The listing builds one solid part. Answer for the finished solid, in the listing's coordinates (mm). A direction names the side the tool comes from. Give positions to 0.01 mm unless a question says otherwise; leave off trailing zeros. Write each loop counter-clockwise with the first axis right and the second up, starting at its lowest first coordinate (ties: lowest second). Pieces come first, ordered by that corner, then holes.
```python
from build123d import *

# Parameters (mm, degrees)
ESQUISSE1_R             = 6.75
ESQUISSE1_R_2           = 15
BOSS_EXTRU_1_DEPTH      = 10
ENL_V_MAT_EXTRU_1_DEPTH = 10
CHANFREIN1_SIZE         = 40


with BuildPart() as part:
    # Esquisse1 → Boss.-Extru.1 (new body)
    with BuildSketch(Plane(origin=(0, 0, 0), x_dir=(1, 0, 0), z_dir=(0, 1, 0))):
        Polygon((0, 0), (0, 250), (240, 250), (320, 250), (560, 250), (640, 250), (880, 250), (880, 0), (880, -140), (780, -140), (780, -130), (620, -130), (620, -140), (520, -140), (520, -130), (360, -130), (360, -140), (260, -140), (260, -130), (100, -130), (100, -140), (0, -140), align=None)
        with Locations(Location((480, 20, 0), (0, 0, 270))):
            Circle(ESQUISSE1_R, mode=Mode.SUBTRACT)
        with Locations(Location((400, 20, 0), (0, 0, 270))):
            Circle(ESQUISSE1_R, mode=Mode.SUBTRACT)
        with Locations(Location((400, 80, 0), (0, 0, 270))):
            Circle(ESQUISSE1_R, mode=Mode.SUBTRACT)
        with Locations(Location((480, 80, 0), (0, 0, 270))):
            Circle(ESQUISSE1_R, mode=Mode.SUBTRACT)
        with Locations(Location((280, 190, 0), (0, 0, 270))):
            Circle(ESQUISSE1_R_2, mode=Mode.SUBTRACT)
        with Locations(Location((600, 190, 0), (0, 0, 270))):
            Circle(ESQUISSE1_R_2, mode=Mode.SUBTRACT)
    extrude(amount=BOSS_EXTRU_1_DEPTH)

    # Esquisse2 → Enlèv. mat.-Extru.1 (cut)
    with BuildSketch(Plane(origin=(0, 10, 0), x_dir=(1, 0, 0), z_dir=(0, 1, 0))):
        Polygon((800, 130), (600, 130), (560, 90), (560, -50), (580, -70), (800, -70), (820, -50), (820, 110), align=None)
        Polygon((80, 130), (60, 110), (60, -50), (80, -70), (300, -70), (320, -50), (320, 90), (280, 130), align=None)
    extrude(amount=-ENL_V_MAT_EXTRU_1_DEPTH, mode=Mode.SUBTRACT)

    # Chanfrein1
    chanfrein1_edges = [part.edges().sort_by_distance(p)[0] for p in [
        (0, 5, -250),
        (880, 5, -250),
    ]]
    chamfer(chanfrein1_edges, length=CHANFREIN1_SIZE)


solid = part.part
```
Item 1: A cutting plane is placed at C-C, the plane y = 5.25. Count the separate pieces of the cut face and the enclosed holes in it, plus the area to 3 significant figures.
Conclusion:
separate pieces: 1
enclosed holes: 8
area: 234,000 mm2
Item 2: Determine the mould class of faces 3 (the face through (300, 5, -110)), 4 (the face through (446, 0, -58)), 5 (the face through (20, 5, -230)), 6 (the face through (860, 5, -230)) for opening direction X: pulls with the +X half, pulls with the -X half, needs draft (parallel to the pull), parting line crosses it, or undercut.
Conclusion:
face 3: undercut
face 4: needs draft
face 5: pulls with the -X half
face 6: pulls with the +X half
Item 3: A cutting plane is placed at B-B, the plane z = -190. Give the vertices of the cut face in (x, y).
Conclusion:
outline: (0, 0) - (265, 0) - (265, 10) - (0, 10) - close; (295, 0) - (585, 0) - (585, 10) - (295, 10) - close; (615, 0) - (880, 0) - (880, 10) - (615, 10) - close
Item 4: Which of the six approach directions +Z, -Z, +X, -X, +Y, -Y give full straight-line access (tool end or side, diameter ignored) to faces 1 (the face through (570, 5, 60)), 2 (the face through (446, 10, -58))?
Conclusion:
face 1: +Y, -Y
face 2: +Z, -Z, +X, -X, +Y
Item 5: A cutting plane is placed at D-D, the plane z = -61. Give the vertices of the cut face in (x, y).
Conclusion:
outline: (0, 0) - (60, 0) - (60, 10) - (0, 10) - close; (320, 0) - (560, 0) - (560, 10) - (320, 10) - close; (820, 0) - (880, 0) - (880, 10) - (820, 10) - close
Item 6: Consider probe 1 along X at (y, z) = (7, -80); probe 2 along X at (y, z) = (9.5, -189); probe 3 along Z at (x, y) = (480, 3). Determine where each line is inside the solid, lowest interval first.
Conclusion:
probe 1: x = 0 to 60, 320 to 393.25, 406.75 to 473.25, 486.75 to 560, 820 to 880
probe 2: x = 0 to 265.03, 294.97 to 585.03, 614.97 to 880
probe 3: z = -250 to -86.75, -73.25 to -26.75, -13.25 to 130
Item 7: A cutting plane is placed at A-A, the plane x = 156. Give the vertices of the cut face in (y, z), plus the area to 3 significant figures.
Conclusion:
outline: (0, -250) - (10, -250) - (10, -130) - (0, -130) - close; (0, 70) - (10, 70) - (10, 130) - (0, 130) - close
area: 1,800 mm2
